from build123d import *

# Parameters (mm, degrees)
SKETCH2_R           = 2.54
SKETCH2_R_2         = 14.3002
BOSS_EXTRUDE1_DEPTH = 3.175


with BuildPart() as part:
    # Sketch2 → Boss-Extrude1 (new body)
    with BuildSketch(Plane.XY):
        Polygon((-77.453506494, 2.582095372), (-77.453506494, -48.217904628), (108.404918235, -48.217904628), (272.064065773, 116.132232758), (236.067449331, 151.977505873), (87.646493506, 2.929897795), align=None)
        with Locations((-21.461195034, -3.501292029)):
            Circle(SKETCH2_R, mode=Mode.SUBTRACT)
        with Locations((-21.461195034, -16.201292029)):
            Circle(SKETCH2_R, mode=Mode.SUBTRACT)
        with Locations((-21.461195034, -28.901292029)):
            Circle(SKETCH2_R, mode=Mode.SUBTRACT)
        with Locations((-21.461195034, -41.601292029)):
            Circle(SKETCH2_R, mode=Mode.SUBTRACT)
        with Locations((-8.761195034, -41.601292029)):
            Circle(SKETCH2_R, mode=Mode.SUBTRACT)
        with Locations((3.938804966, -41.601292029)):
            Circle(SKETCH2_R, mode=Mode.SUBTRACT)
        with Locations((16.638804966, -41.601292029)):
            Circle(SKETCH2_R, mode=Mode.SUBTRACT)
        with Locations((29.338804966, -41.601292029)):
            Circle(SKETCH2_R, mode=Mode.SUBTRACT)
        with Locations((42.038804966, -41.601292029)):
            Circle(SKETCH2_R, mode=Mode.SUBTRACT)
        with Locations((-8.761195034, -3.501292029)):
            Circle(SKETCH2_R, mode=Mode.SUBTRACT)
        with Locations((3.938804966, -3.501292029)):
            Circle(SKETCH2_R, mode=Mode.SUBTRACT)
        with Locations((16.638804966, -3.501292029)):
            Circle(SKETCH2_R, mode=Mode.SUBTRACT)
        with Locations((29.338804966, -3.501292029)):
            Circle(SKETCH2_R, mode=Mode.SUBTRACT)
        with Locations((42.038804966, -3.501292029)):
            Circle(SKETCH2_R, mode=Mode.SUBTRACT)
        with Locations((54.738804966, -3.501292029)):
            Circle(SKETCH2_R, mode=Mode.SUBTRACT)
        with Locations((67.438804966, -3.501292029)):
            Circle(SKETCH2_R, mode=Mode.SUBTRACT)
        with Locations((80.138804966, -3.501292029)):
            Circle(SKETCH2_R, mode=Mode.SUBTRACT)
        with Locations((92.838804966, -3.501292029)):
            Circle(SKETCH2_R, mode=Mode.SUBTRACT)
        with Locations((92.838804966, -16.201292029)):
            Circle(SKETCH2_R, mode=Mode.SUBTRACT)
        with Locations((92.838804966, -28.901292029)):
            Circle(SKETCH2_R, mode=Mode.SUBTRACT)
        with Locations((54.738804966, -41.601292029)):
            Circle(SKETCH2_R, mode=Mode.SUBTRACT)
        with Locations((67.438804966, -41.601292029)):
            Circle(SKETCH2_R, mode=Mode.SUBTRACT)
        with Locations((80.138804966, -41.601292029)):
            Circle(SKETCH2_R, mode=Mode.SUBTRACT)
        with Locations((92.838804966, -41.601292029)):
            Circle(SKETCH2_R, mode=Mode.SUBTRACT)
        with Locations((69.080846726, -22.817904628)):
            Circle(SKETCH2_R_2, mode=Mode.SUBTRACT)
        with Locations((35.310660441, -22.817904628)):
            Circle(SKETCH2_R_2, mode=Mode.SUBTRACT)
        with Locations((1.237019836, -22.817904628)):
            Circle(SKETCH2_R_2, mode=Mode.SUBTRACT)
        with Locations((-52.827339559, -22.817904628)):
            Circle(SKETCH2_R_2, mode=Mode.SUBTRACT)
        with Locations((136.992213353, 16.487025642)):
            Circle(SKETCH2_R, mode=Mode.SUBTRACT)
        with Locations((145.953531631, 25.486179753)):
            Circle(SKETCH2_R, mode=Mode.SUBTRACT)
        with Locations((154.91484991, 34.485333864)):
            Circle(SKETCH2_R, mode=Mode.SUBTRACT)
        with Locations((163.876168189, 43.484487974)):
            Circle(SKETCH2_R, mode=Mode.SUBTRACT)
        with Locations((172.837486468, 52.483642085)):
            Circle(SKETCH2_R, mode=Mode.SUBTRACT)
        with Locations((181.798804747, 61.482796195)):
            Circle(SKETCH2_R, mode=Mode.SUBTRACT)
        with Locations((190.760123026, 70.481950306)):
            Circle(SKETCH2_R, mode=Mode.SUBTRACT)
        with Locations((199.721441305, 79.481104416)):
            Circle(SKETCH2_R, mode=Mode.SUBTRACT)
    extrude(amount=BOSS_EXTRUDE1_DEPTH)


solid = part.part
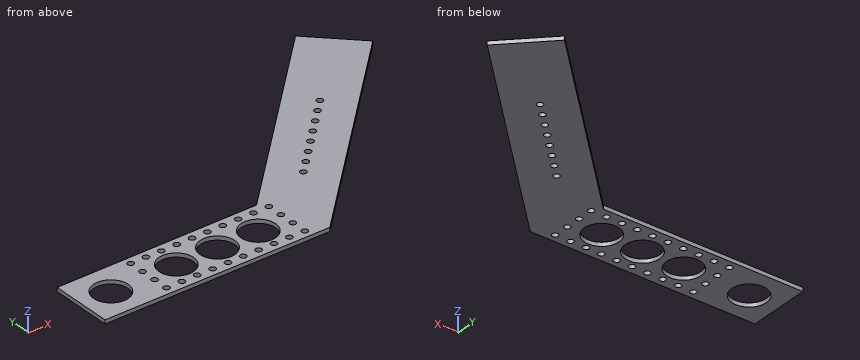
Read the model definition and answer for the solid it produces. Units are mm, in the model's axes. Give positions to 0.01 mm unless a question says otherwise; leave off trailing zeros. Write each loop counter-clockwise with the first axis right and the second up, starting at its lowest first coordinate (ties: lowest second). Pieces come first, ordered by that corner, then holes. Notation, with made-up numbers: (70.5, 57.5) - (120.5, 57.5) arc R14 ccw to (120.5, 63.5) - close; hole circle Ø2 at (0, 86). An arc over 180 degrees is marked (long way). Answer in a Markdown table with one row per item. Add a question column.
Item 1: Find the intervals of material crossed by L1, parallel to Y at x = 43, z = 0.3; L2, parallel to Y at x = 92.5, z = 0.8; L3, parallel to Y at x = 30, z = 2.2, in increasing order.
Item 2: Section C-C, the plane x = 123 is taken. Write down the section's boundary in (y, z) (3 decimals).
Item 3: Section B-B, the plane y = 137.5 is taken. Write down the section's boundary in (x, z) (3 decimals), and give its area (3 significant figures).
Item 4: Flat-ended cylindrical pins translate along their axes: P1, Ø4, axis at x = -8.76, y = -3.5, coming from the +Z side; P2, Ø1, axis at y = 13, z = 2, coming from the +X side; P3, Ø6, axis at x = -21.46, y = -16.2, coming from the +Z side (3 decimals). Find the tip coordinate at first contact, or state that the pin passes through.
Item 5: Section A-A, the plane z = 0.6 is taken. Count the separate pieces of the cut face and the enclosed holes in it, and give its area (3 significant figures).
Recorded:
| question | item | result |
|---|---|---|
| 1 | L1 | y = -48.22 to -43.95, -39.25 to -34.87, -10.76 to -5.85, -1.15 to 2.84 |
| 1 | L2 | y = -48.22 to -44.12, -39.08 to -31.42, -26.38 to -18.72, -13.68 to -6.02, -0.98 to 7.8 |
| 1 | L3 | y = -48.22 to -44.05, -39.15 to -36.1, -9.54 to -5.95, -1.05 to 2.81 |
| 2 | outline | (-33.561, 0) - (38.433, 0) - (38.433, 3.175) - (-33.561, 3.175) - close |
| 3 | outline | (221.651, 0) - (250.606, 0) - (250.606, 3.175) - (221.651, 3.175) - close |
| 3 | area | 91.9 mm2 |
| 4 | P1 | passes through |
| 4 | P2 | stops at x = 169.86 |
| 4 | P3 | stops at z = 3.175 |
| 5 | separate pieces | 1 |
| 5 | enclosed holes | 36 |
| 5 | area | 17,000 mm2 |
